from build123d import *

# Parameters (mm, degrees)
SKETCH1_W           = 50.8
SKETCH1_H           = 22.86
BOSS_EXTRUDE1_DEPTH = 1.5875
SKETCH2_W           = 6.35
SKETCH2_H           = 15.875
BOSS_EXTRUDE2_DEPTH = 12.7
SKETCH3_W           = 22.225
SKETCH3_H           = 14.2875
BOSS_EXTRUDE3_DEPTH = 19.05
SKETCH4_W           = 12.7
SKETCH4_H           = 3.175
BOSS_EXTRUDE4_DEPTH = 9.525
SKETCH5_R           = 1.27
CUT_EXTRUDE1_DEPTH  = 34.744738849


with BuildPart() as part:
    # Sketch1 → Boss-Extrude1 (new body)
    with BuildSketch(Plane(origin=(0, 0, 0), x_dir=(1, 0, 0), z_dir=(0, 1, 0))):
        Rectangle(SKETCH1_W, SKETCH1_H)
    extrude(amount=BOSS_EXTRUDE1_DEPTH)

    # Sketch2 → Boss-Extrude2 (add)
    with BuildSketch(Plane(origin=(0, 1.5875, 0), x_dir=(1, 0, 0), z_dir=(0, 1, 0))):
        with Locations((-22.225, 0)):
            Rectangle(SKETCH2_W, SKETCH2_H)
    extrude(amount=BOSS_EXTRUDE2_DEPTH)

    # Sketch3 → Boss-Extrude3 (add)
    with BuildSketch(Plane(origin=(0, 1.5875, 0), x_dir=(1, 0, 0), z_dir=(0, 1, 0))):
        with Locations((-7.9375, 0)):
            Rectangle(SKETCH3_W, SKETCH3_H)
    extrude(amount=BOSS_EXTRUDE3_DEPTH)

    # Sketch4 → Boss-Extrude4 (add)
    with BuildSketch(Plane(origin=(0, 1.5875, 0), x_dir=(1, 0, 0), z_dir=(0, 1, 0))):
        with Locations((11.719402779, 9.8425)):
            Rectangle(SKETCH4_W, SKETCH4_H)
    extrude(amount=BOSS_EXTRUDE4_DEPTH)

    # Sketch5 → Cut-Extrude1 (cut, through all)
    with BuildSketch(Plane(origin=(0, 1.5875, 0), x_dir=(1, 0, 0), z_dir=(0, 1, 0))):
        with Locations(Location((-22.86, 8.89, 0), (0, 0, 270))):
            Circle(SKETCH5_R)
        with Locations(Location((22.86, 8.89, 0), (0, 0, 270))):
            Circle(SKETCH5_R)
        with Locations(Location((-22.86, -8.89, 0), (0, 0, 270))):
            Circle(SKETCH5_R)
        with Locations(Location((22.86, -8.89, 0), (0, 0, 270))):
            Circle(SKETCH5_R)
    extrude(amount=-CUT_EXTRUDE1_DEPTH, mode=Mode.SUBTRACT)


solid = part.part
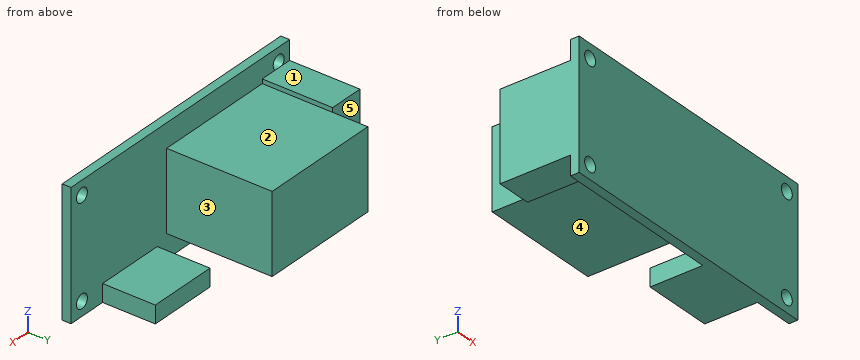
Verification items for the finished model (mm, model axes). Face numbers are marked on the shaded views. A direction names the side the tool comes from. Coordinates: 2 decimals unless noted, no trailing zeros. Order: outer loops, then holes, each group sorted by start corner. A loop starts at its lowest first (then second) coordinate and runs counter-clockwise, first axis right, second up. Notation, with made-up numbers: (-13, 73) -> (40, 73) arc R18 cw to (40, 97) -> close; hole circle Ø6 at (72.5, -32). An arc over 180 degrees is marked (long way). Put each result on its own line as item: value. Start each with the question number.
1. Cross-section at C-C, the plane x = 22.86. Record the boundary of the cut face in (y, z).
2. Cross-section at B-B, the plane z = -8.89. Record the boundary of the cut face in (x, y), then the cut area to 3 significant figures.
3. Go/stop test with flat-tipped pins: pin 1 Ø1.9 at (x, z) = (-23.5, 2.5) entering from +Y; pin 2 Ø6 at (y, z) = (6, -3) entering from +X (3 decimals); pin 3 Ø9.5 at (x, y) = (-7, 15) entering from +Z; pin 4 Ø2 at (x, z) = (22.86, 8.89) entering from +Y. Record where each tip stops, or that it passes through.
4. Material ranges on L1, parallel to X at y = 0.9, z = -8.89; L2, parallel to X at y = 15.25, z = -3.75 (3 decimals); L3, parallel to Y at x = 7, z = -4, recorded low to high. Write a range as [from, to].
5. Access from +Z, -Z, +X, -X, +Y, -Y to the whole of each face (thin tool, end or side, straight path). Record for the marked faces 1, 2, 3, 4 and 5.
Computed:
1. outline: (0, -11.43) -> (1.59, -11.43) -> (1.59, -10.16) -> (0, -10.16) -> close; (0, -7.62) -> (1.59, -7.62) -> (1.59, 7.62) -> (0, 7.62) -> close; (0, 10.16) -> (1.59, 10.16) -> (1.59, 11.43) -> (0, 11.43) -> close
2. outline: (-25.4, 0) -> (-24.13, 0) -> (-24.13, 1.59) -> (-25.4, 1.59) -> close; (-21.59, 0) -> (21.59, 0) -> (21.59, 1.59) -> (18.07, 1.59) -> (18.07, 11.11) -> (5.37, 11.11) -> (5.37, 1.59) -> (-21.59, 1.59) -> close; (24.13, 0) -> (25.4, 0) -> (25.4, 1.59) -> (24.13, 1.59) -> close
2. area: 194 mm2
3. pin 1: y = 14.29
3. pin 2: x = 3.175
3. pin 3: z = 7.14
3. pin 4: through
4. L1: [-25.4, -24.13], [-21.59, 21.59], [24.13, 25.4]
4. L2: [-19.05, 3.175]
4. L3: [0, 1.59]
5. face 1: +Z, +X, -X, +Y
5. face 2: +Z, +X, +Y
5. face 3: +Z, -Z, +X, +Y
5. face 4: -Z, +X, +Y
5. face 5: +Z, -Z, -X, +Y
